The drawing under review shows one solid part. Ordinate dimensions are in mm from its lowest x, y, z. Round coordinates to 2 decimals unless told otherwise and drop trailing zeros. Order: outer loops, then holes, each group sorted by start corner. A loop starts at its lowest first (then second) coordinate and runs counter-clockwise, first axis right, second up. Notation, with made-up numbers: M 39,24.5 L 43,24.5 A27 cw 43,45.5 Z; hole C 43.5,-6 d7. An arc over 180 degrees is marked long. Write item = value, one per line. Start each with the question number.
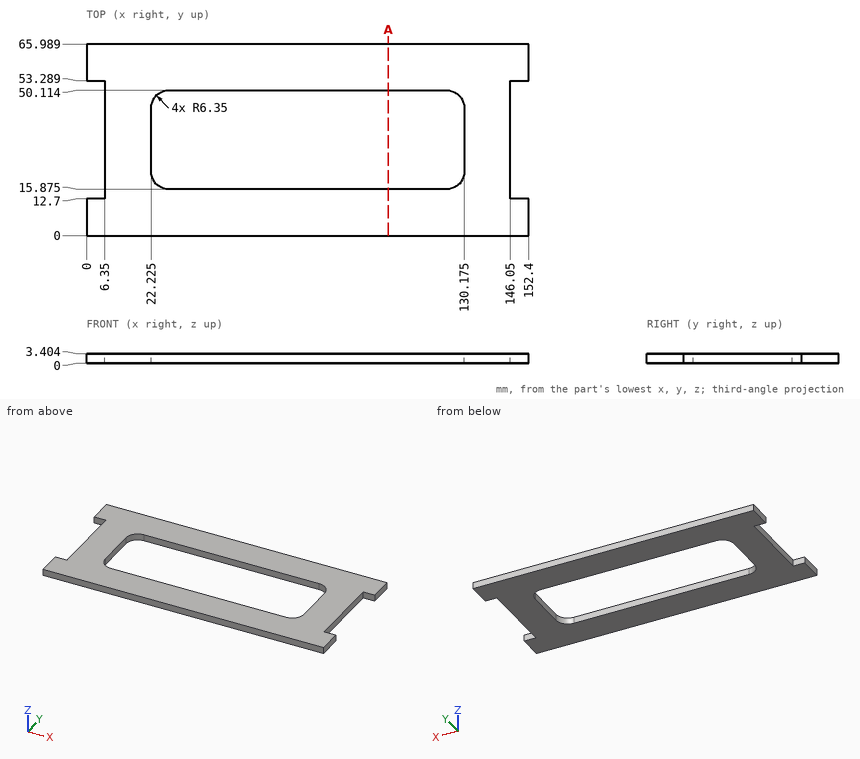
(1) For line 1 along Y through (x, z) = (51.5, 1.7) (1 decimal); line 2 along X through (y, z) = (20, 0.4); line 3 along X through (y, z) = (49.5, 0.35), list the stretches that pass through material, from the lowest coordinate up. Write a range as [from, to].
(2) Consider section A-A, the plane x = 104. Write out the cut boundary in (y, z) (1 decimal), then the cut area to 3 significant figures.
(3) Insertion check: pin 1 (1.7 mm diameter, centred on y = 36, z = 2.5, fed in from -X); pin 2 (1 mm diameter, centred on x = 2.5, z = 1, fed in from -Y); pin 3 (1.5 mm diameter, centred on y = 38, z = 0.5, fed in from +X). Each pin has a flat end and moves straight along its axis. Give the tip position at first contact, or say it passes through.
Completed:
q1.line_1 = [0, 15.9], [50.1, 66]
q1.line_2 = [6.35, 22.63], [129.77, 146.05]
q1.line_3 = [6.35, 25.85], [126.55, 146.05]
q2.outline = M 0,0 L 15.9,0 L 15.9,3.4 L 0,3.4 Z; M 50.1,0 L 66,0 L 66,3.4 L 50.1,3.4 Z
q2.area = 108 mm2
q3.pin_1 = 6.35
q3.pin_2 = 0
q3.pin_3 = 146.05
